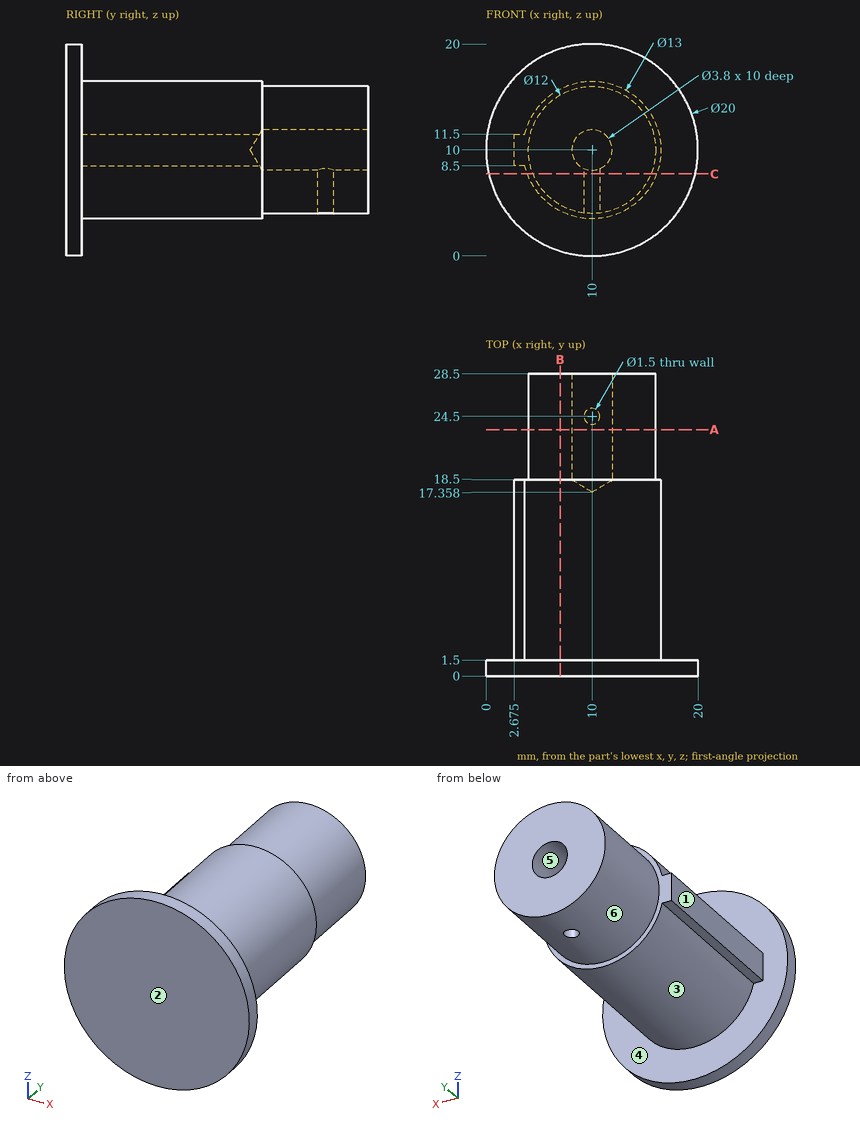
Design review of the part shown in the three views and the two pictorial views. Dimensions are in mm from the part's minimum x, y and z. A direction names the side the tool comes from. Give positions to 0.01 mm unless a question says otherwise; leave off trailing zeros. Loops run counter-clockwise (first coordinate to the right, second up) from the corner with the lowest first, then second, coordinate; pieces in that order, holes last. Notation, with made-up numbers: M -8.75,36.5 L 11.25,36.5 A11 cw 11.25,45.5 Z; hole C -36,82 d5. An arc over 180 degrees is marked long. Answer as a JSON object with one key per item and string values. Group by question number.
Q1. Insertion check: P1, Ø5, axis at y = 14, z = 13.5, coming from the +X side; P2, Ø3.5, axis at y = 6, z = 9.5, coming from the -X side (1 decimal); P3, Ø6, axis at y = 17.5, z = 18, coming from the +X side (1 decimal). Each pin has a flat end and moves straight along its axis. Give the tip position at first contact, or say it passes through.
Q2. Add section B-B on x = 7. Give the boundary of the cut face in (y, z).
Q3. Tool access review of the marked faces 1, 2 and 3: name each direction out of +Z, -Z, +X, -X, +Y, -Y from which nothing blocks a thin tool from reaching the whole face with its end or side.
Q4. Add section C-C on z = 7.75. Give the boundary of the cut face in (x, y).
Q5. Add section A-A on y = 23.25. Give the boundary of the cut face in (x, z), and give its area (3 significant figures).
Q6. For probe 1 along Z at (x, y) = (10, 26.5); probe 2 along Y at (x, z) = (3.5, 16.75), list the stretches that pass through material, from the lowest coordinate up. Write a range as [from, to].
Q7. Mouldability with a two-part tool opening along Z and no side actions: class the marked faces 4, 5 and 6 as +Z half, -Z half, draft (parallel to the pull), parting line (faces both ways), or undercut.
Checked values:
{
 "1": {"P1": "x = 16.42", "P2": "x = 2.7", "P3": "x = 14.2"},
 "2": {"outline": "M 0,0.46 L 1.5,0.46 L 1.5,4.23 L 18.5,4.23 L 18.5,4.8 L 28.5,4.8 L 28.5,15.2 L 18.5,15.2 L 18.5,15.77 L 1.5,15.77 L 1.5,19.54 L 0,19.54 Z"},
 "3": {"face 1": "+Z, -Z, -X, +Y", "face 2": "+Z, -Z, +X, -X, -Y", "face 3": "+Y"},
 "4": {"outline": "M 0.26,0 L 19.74,0 L 19.74,1.5 L 16.1,1.5 L 16.1,18.5 L 15.56,18.5 L 15.56,28.5 L 4.44,28.5 L 4.44,18.5 L 3.9,18.5 L 3.9,1.5 L 0.26,1.5 Z; hole C 10,24.5 d1.5"},
 "5": {"outline": "C 10,10 d12; hole C 10,10 d3.8", "area": "102 mm²"},
 "6": {"probe 1": "[4, 8.1], [11.9, 16]", "probe 2": "[0, 1.5]"},
 "7": {"face 4": "draft", "face 5": "undercut", "face 6": "parting line"}
}
